Could you check a few things on this drawing? It's one solid part, dimensions in mm from its lowest x, y, z. A direction names the side the tool comes from. Coordinates: 2 decimals unless noted, no trailing zeros. Write each loop counter-clockwise with the first axis right and the second up, starting at its lowest first coordinate (ties: lowest second). Pieces come first, ordered by that corner, then holes. Notation, with made-up numbers: M 18.25,-19.5 L 33.25,-19.5 A13 cw 33.25,0.5 Z; hole C 84,32 d7. An arc over 180 degrees is marked long. Use a Markdown table: item, result.
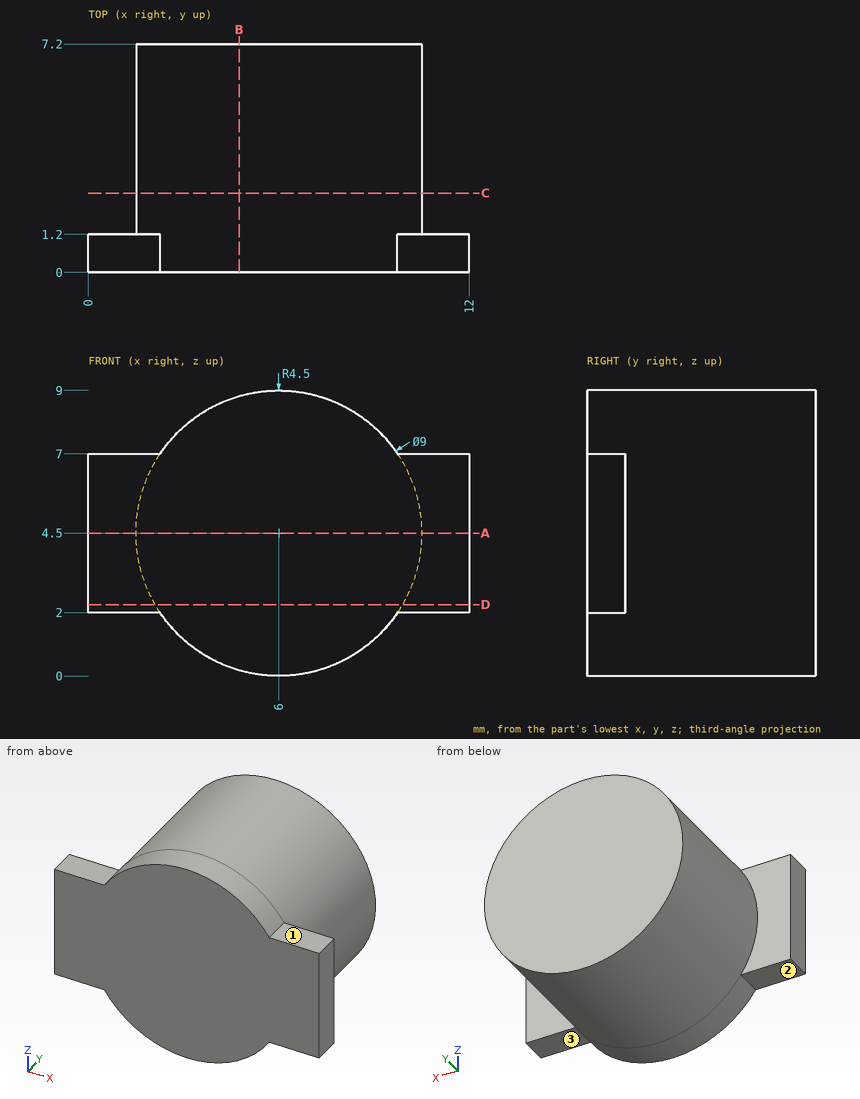
1. Will these pins go through, and if not, where does the flat tip stop? pin 1 Ø1.1 at (x, z) = (11.5, 5) entering from +Y; pin 2 Ø3 at (x, y) = (9.5, 4.5) entering from -Z; pin 3 Ø4 at (y, z) = (5.5, 4) entering from -X.
Answers follow:
| item | result |
|---|---|
| pin 1 | stops at y = 1.2 |
| pin 2 | stops at z = 0.47 |
| pin 3 | stops at x = 1.5 |
2. Suppose I cut it at A-A on z = 4.5. Write out the boundary of the cut face in (x, y).
Answers follow:
| item | result |
|---|---|
| outline | M 0,0 L 12,0 L 12,1.2 L 10.5,1.2 L 10.5,7.2 L 1.5,7.2 L 1.5,1.2 L 0,1.2 Z |
3. Which directions (+Z, -Z, +X, -X, +Y, -Y) give clear straight access to the entire face, cutting with the end or side of a thin tool? Please do the marked faces 1, 2 and 3.
Answers follow:
| item | result |
|---|---|
| face 1 | +Z, +X, +Y, -Y |
| face 2 | -Z, -X, +Y, -Y |
| face 3 | -Z, +X, +Y, -Y |
4. I need wall thicknesses on probe 1 along Z at (x, y) = (8.75, 2); probe 2 along Y at (x, z) = (0.5, 6); probe 3 along X at (y, z) = (6.75, 4). Which ranges of each line are inside material? Lowest first, please.
Answers follow:
| item | result |
|---|---|
| probe 1 | z = 0.94 to 8.06 |
| probe 2 | y = 0 to 1.2 |
| probe 3 | x = 1.53 to 10.47 |
5. Suppose I cut it at C-C on y = 2.5. Write out the boundary of the cut face in (x, z).
Answers follow:
| item | result |
|---|---|
| outline | C 6,4.5 d9 |
6. Suppose I cut it at B-B on x = 4.75. Write out the boundary of the cut face in (y, z).
Answers follow:
| item | result |
|---|---|
| outline | M 0,0.18 L 7.2,0.18 L 7.2,8.82 L 0,8.82 Z |
7. Suppose I cut it at D-D on z = 2.25. Write out the boundary of the cut face in (x, y).
Answers follow:
| item | result |
|---|---|
| outline | M 0,0 L 12,0 L 12,1.2 L 9.9,1.2 L 9.9,7.2 L 2.1,7.2 L 2.1,1.2 L 0,1.2 Z |
